Geometry: final body of the model. Coordinates: model frame, mm. A direction names the side the tool comes from. Round coordinates to 2 decimals unless told otherwise and drop trailing zeros. Write each loop counter-clockwise with the first axis right and the second up, starting at its lowest first coordinate (ties: lowest second). Pieces come first, ordered by that corner, then holes. Notation, with made-up numbers: M 5,16 L 26,16 A32 cw 26,47 Z; hole C 87,41 d3. An arc over 180 degrees is marked long. Answer as CSV lines item,"result". Start each with the question number.
Q1. Reachability of faces 1 (the cylindrical face through (8.554, -0.23, 4.46)), 2 (the flat face through (8, -1, 3.7)), 3 (the flat face through (4.5, 2, 4)) from +Z, -Z, +X, -X, +Y, -Y: full face, straight path, thin tool, end or side. Return the list, or none.
Q2. First-contact query: pin 1 (1.6 mm diameter, centred on x = -8, y = 0, fed in from -Z); pin 2 (0.5 mm diameter, centred on y = -1.5, z = 3, fed in from -X); pin 3 (1.7 mm diameter, centred on y = 1.5, z = 3.5, fed in from +X); pin 4 (1.1 mm diameter, centred on y = -0.5, z = 2, fed in from +X). Flat tips, straight axial feed; report the tip coordinate or a pass-through.
Q3. Ray query, probe 1 along X at (y, z) = (1.45, 4.1); probe 2 along Y at (x, z) = (0, 1.6); probe 3 along X at (y, z) = (1.3, 3.15). Return the intervals inside material, ascending.
Q4. Mould query, pull axis Y, two halves, no side actions, for faces 4 (the flat face through (-7, 0, 5.2)), 5 (the flat face through (0, 2.5, 1)), 6 (the cylindrical face through (0.108, -0.488, 0.986)), 7 (the flat face through (0, -2.5, 1)). Classes: pulls with the +Y half, pulls with the -Y half, needs draft (parallel to the pull), parting line crosses it, or undercut.
Q5. Section query B-B on x = 8. Output: boundary loops of the cut face in (y, z).
Q6. Section query C-C on z = 4.55. Output: boundary loops of the cut face in (x, y).
Q7. Section query D-D on z = 0.65. Output: boundary loops of the cut face in (x, y).
Q8. Section query A-A on z = 2.9. Output: boundary loops of the cut face in (x, y), and give its area (3 significant figures).
```python
from build123d import *

# Parameters (mm, degrees)
SKETCH_1_R      = 0.5
EXTRUDE_1_DEPTH = 2
EXTRUDE_2_DEPTH = 5.2
EXTRUDE_START   = 5.2
SKETCH_1_13_W   = 3
SKETCH_1_13_H   = 5
SKETCH_1_13_R   = 0.6
EXTRUDE_3_DEPTH = 1.5


with BuildPart() as part:
    # 草图1 → 凸台-拉伸1 (new body)
    with BuildSketch(Plane.XY):
        with BuildLine():
            Line((4.5, 2.5), (-4.5, 2.5))
            Line((-4.5, 2.5), (-4.5, 0.953939201))
            ThreePointArc((-4.5, 0.953939201), (-3.608392022, 0.806225775), (-3.2, 0))
            ThreePointArc((-3.2, 0), (-3.608392022, -0.806225775), (-4.5, -0.953939201))
            Line((-4.5, -0.953939201), (-4.5, -2.5))
            Line((-4.5, -2.5), (4.5, -2.5))
            Line((4.5, -2.5), (4.5, -0.953939201))
            ThreePointArc((4.5, -0.953939201), (3.2, 0), (4.5, 0.953939201))
            Line((4.5, 0.953939201), (4.5, 2.5))
        make_face()
        with BuildLine():
            ThreePointArc((2.5, 0), (2, -0.5), (1.5, 0))
            ThreePointArc((1.5, 0), (2, 0.5), (2.5, 0))
        make_face(mode=Mode.SUBTRACT)
        with Locations((-2, 0)):
            Circle(SKETCH_1_R, mode=Mode.SUBTRACT)
        with BuildLine():
            ThreePointArc((0.5, 0), (0, -0.5), (-0.5, 0))
            ThreePointArc((-0.5, 0), (0, 0.5), (0.5, 0))
        make_face(mode=Mode.SUBTRACT)
    extrude(amount=EXTRUDE_1_DEPTH)

    # 草图1<10> → 凸台-拉伸2 (add)
    with BuildSketch(Plane.XY):
        with BuildLine():
            Line((-4.5, 0.953939201), (-4.5, 2.5))
            Line((-4.5, 2.5), (-6.5, 2.5))
            Line((-6.5, 2.5), (-6.5, -2.5))
            Line((-6.5, -2.5), (-4.5, -2.5))
            Line((-4.5, -2.5), (-4.5, -0.953939201))
            ThreePointArc((-4.5, -0.953939201), (-5.2, 0), (-4.5, 0.953939201))
        make_face()
        with BuildLine():
            Line((6.5, 2.5), (4.5, 2.5))
            Line((4.5, 2.5), (4.5, 0.953939201))
            ThreePointArc((4.5, 0.953939201), (5.2, 0), (4.5, -0.953939201))
            Line((4.5, -0.953939201), (4.5, -2.5))
            Line((4.5, -2.5), (6.5, -2.5))
            Line((6.5, -2.5), (6.5, 2.5))
        make_face()
    extrude(amount=EXTRUDE_2_DEPTH)

    # 草图1<13> → 凸台-拉伸3 (add)
    # profile 1 of 2: a face of its own
    with BuildSketch(Plane.XY.offset(EXTRUDE_START)):
        with Locations((-8, 0)):
            Rectangle(SKETCH_1_13_W, SKETCH_1_13_H)
        with Locations((-8, 0)):
            Circle(SKETCH_1_13_R, mode=Mode.SUBTRACT)
    # profile 2 of 2: a face of its own
    with BuildSketch(Plane.XY.offset(EXTRUDE_START)):
        with Locations((8, 0)):
            Rectangle(SKETCH_1_13_W, SKETCH_1_13_H)
        with Locations((8, 0)):
            Circle(SKETCH_1_13_R, mode=Mode.SUBTRACT)
    extrude(amount=-EXTRUDE_3_DEPTH)


solid = part.part
```
Entries:
1,face 1,"+Z, -Z"
1,face 2,"-Z, +X, +Y, -Y"
1,face 3,"+Z, +Y, -Y"
2,pin 1,"stops at z = 3.7"
2,pin 2,"stops at x = -6.5"
2,pin 3,"stops at x = 9.5"
2,pin 4,"stops at x = 6.5"
3,probe 1,"x = -9.5 to -4.5, 4.5 to 9.5"
3,probe 2,"y = -2.5 to -0.5, 0.5 to 2.5"
3,probe 3,"x = -6.5 to -4.5, 4.5 to 6.5"
4,face 4,"needs draft"
4,face 5,"pulls with the +Y half"
4,face 6,"undercut"
4,face 7,"pulls with the -Y half"
5,outline,"M -2.5,3.7 L -0.6,3.7 L -0.6,5.2 L -2.5,5.2 Z; M 0.6,3.7 L 2.5,3.7 L 2.5,5.2 L 0.6,5.2 Z"
6,outline,"M -9.5,-2.5 L -4.5,-2.5 L -4.5,-0.95 A1 cw -4.5,0.95 L -4.5,2.5 L -9.5,2.5 Z; M 4.5,-2.5 L 9.5,-2.5 L 9.5,2.5 L 4.5,2.5 L 4.5,0.95 A1 cw 4.5,-0.95 Z; hole C -8,0 d1.2; hole C 8,0 d1.2"
7,outline,"M -6.5,-2.5 L 6.5,-2.5 L 6.5,2.5 L -6.5,2.5 Z; hole C -4.2,0 d2; hole C -2,0 d1; hole C 0,0 d1; hole C 2,0 d1; hole C 4.2,0 d2"
8,outline,"M -6.5,-2.5 L -4.5,-2.5 L -4.5,-0.95 A1 cw -4.5,0.95 L -4.5,2.5 L -6.5,2.5 Z; M 4.5,-2.5 L 6.5,-2.5 L 6.5,2.5 L 4.5,2.5 L 4.5,0.95 A1 cw 4.5,-0.95 Z"
8,area,"18.0 mm^2"
